Input: part model. Units: mm. Frame: model coordinates. A direction names the side the tool comes from. Round coordinates to 2 decimals unless told otherwise and drop trailing zeros. Write each loop counter-clockwise with the first axis right and the second up, starting at its lowest first coordinate (ties: lowest second). Pieces come first, ordered by that corner, then holes. Notation, with made-up numbers: M 43,17 L 92,17 A5 cw 92,25 Z; hole C 72,12.25 d2. An arc over 180 degrees is marked long. Use one line per item in the form item = value. Start each with the question number.
Autodesk Inventor part; units mm, degrees
ref_plane "YZ Plane" through (0, 0, 0) normal (1, 0, 0) x (0, 1, 0)
ref_plane "XZ Plane" through (0, 0, 0) normal (0, 1, 0) x (-1, 0, 0)
ref_plane "XY Plane" through (0, 0, 0) normal (0, 0, 1) x (1, 0, 0)
sketch "Sketch1" plane through (0, 0, 0) normal (0, 1, 0) x (-1, 0, 0)
  line L0 (71, -11.5) -> (-71, -11.5)
  line L1 (-71, -11.5) -> (-71, 11.5)
  line L2 (-71, 11.5) -> (71, 11.5)
  line L3 (71, 11.5) -> (71, -11.5)
  line L4 (68, -11.5) -> (68, 11.5)
  line L5 (48.5, -14.5) -> (28.5, -14.5)
  line L6 (28.5, -14.5) -> (28.5, -11.5)
  line L7 (28.5, -11.5) -> (48.5, -11.5)
  line L8 (48.5, -11.5) -> (48.5, -14.5)
  line L9 (48.5, 11.5) -> (28.5, 11.5)
  line L10 (28.5, 11.5) -> (28.5, 14.5)
  line L11 (28.5, 14.5) -> (48.5, 14.5)
  line L12 (48.5, 14.5) -> (48.5, 11.5)
  line L13 (38.5, -14.5) -> (38.5, -11.5) construction
  line L14 (-48.5, -14.5) -> (-48.5, -11.5)
  line L15 (-38.5, -14.5) -> (-38.5, -11.5) construction
  line L16 (-48.5, -11.5) -> (-28.5, -11.5)
  line L17 (-28.5, 11.5) -> (-48.5, 11.5)
  line L18 (-28.5, -14.5) -> (-48.5, -14.5)
  line L19 (-48.5, 14.5) -> (-28.5, 14.5)
  line L20 (-28.5, 14.5) -> (-28.5, 11.5)
  line L21 (-28.5, -11.5) -> (-28.5, -14.5)
  line L22 (-48.5, 11.5) -> (-48.5, 14.5)
  point P0 (0, 0)
  point P1 (-71, 0)
  point P2 (0, -11.5)
  point P3 (48.5, -11.5)
  point P4 (28.5, -11.5)
  point P5 (-28.5, -11.5)
  point P6 (-48.5, -11.5)
  point P7 (-48.5, 11.5)
  point P8 (-28.5, 11.5)
  point P9 (28.5, 11.5)
  point P10 (48.5, 11.5)
  dimension "d0" = 23
  dimension "d1" = 142
  dimension "d2" = 3
  dimension "d3" = 20
  dimension "d4" = 3
  dimension "d5" = 20
  dimension "d6" = 3
  dimension "d7" = 38.5
  dimension "d10" = 77
extrude "Extrusion1" add sketch "Sketch1" along normal blind 3
equation "\"d0\" = stack"
equation "\"d3\" = finger"
equation "\"d4\" = thickness"
equation "\"d5\" = finger"
equation "\"d15\" = thickness"
equation "\"stack\" = 23"
equation "\"finger\" = 20"
equation "\"thickness\" = 3"
properties part number "BungaSign-Bigger-Sides-Right"
Item 1: Ray query, line 1 (Z direction, x = 12.5, y = 0.7). Return the intervals inside material, ascending. Write a range as from..to.
Item 2: Cut plane B-B (x = 51). Output: boundary loops of the cut face in (y, z), plus the area to 3 significant figures.
Item 3: Draft query along X for faces 1 (the face through (28.5, 1, -13)), 2 (the face through (-38, 1, 14.5)), 3 (the face through (-71, 1, 0)), 4 (the face through (48.5, 1, 13)). Return one class per face: +X half, -X half, draft (parallel to the pull), parting line (faces both ways), or undercut.
Item 4: First-contact query: pin 1 (1.5 mm diameter, centred on y = 1, z = -13, fed in from +X); pin 2 (1.5 mm diameter, centred on x = -65, y = 2, fed in from -Z); pin 3 (0.9 mm diameter, centred on x = 64.5, y = 1, fed in from +Z). Flat tips, straight axial feed; report the tip coordinate or a pass-through.
Item 5: Reachability of faces 5 (the face through (0, 1, -11.5)), 6 (the face through (-28.5, 1, 13)), 7 (the face through (-60, 1, 11.5)) from +Z, -Z, +X, -X, +Y, -Y: full face, straight path, thin tool, end or side. Return the list, or none.
Item 6: Cut plane A-A (y = 1.85). Output: boundary loops of the cut face in (x, z), plus the area to 3 significant figures.
Final values:
q1.line_1 = -11.5..11.5
q2.outline = M 0,-11.5 L 3,-11.5 L 3,11.5 L 0,11.5 Z
q2.area = 69.0 mm^2
q3.face_1 = undercut
q3.face_2 = draft
q3.face_3 = -X half
q3.face_4 = +X half
q4.pin_1 = 48.5
q4.pin_2 = -11.5
q4.pin_3 = 11.5
q5.face_5 = -Z, +Y, -Y
q5.face_6 = +Z, +Y, -Y
q5.face_7 = +Z, -X, +Y, -Y
q6.outline = M -71,-11.5 L -48.5,-11.5 L -48.5,-14.5 L -28.5,-14.5 L -28.5,-11.5 L 28.5,-11.5 L 28.5,-14.5 L 48.5,-14.5 L 48.5,-11.5 L 71,-11.5 L 71,11.5 L 48.5,11.5 L 48.5,14.5 L 28.5,14.5 L 28.5,11.5 L -28.5,11.5 L -28.5,14.5 L -48.5,14.5 L -48.5,11.5 L -71,11.5 Z
q6.area = 3,510 mm^2
